Geometry check sheet. Reference: the model listing, model coordinates, mm. A direction names the side the tool comes from. Coordinates: 2 decimals unless noted, no trailing zeros. Order: outer loops, then holes, each group sorted by start corner. A loop starts at its lowest first (then second) coordinate and runs counter-clockwise, first axis right, second up. Notation, with made-up numbers: (-32, -9) - (-19, -9) arc R14 ccw to (-19, -1) - close; hole circle Ø9 at (-29, 78.25). An arc over 180 degrees is marked (long way). One line per item, written item: value. Start each with the question number.
```python
from build123d import *

# Parameters (mm, degrees)
SKETCH1_W           = 125
SKETCH1_H           = 382
BOSS_EXTRUDE1_DEPTH = 2
SKETCH2_W           = 216
SKETCH2_H           = 16
BOSS_EXTRUDE2_DEPTH = 10
SKETCH3_W           = 210
SKETCH3_H           = 10
CUT_EXTRUDE1_DEPTH  = 390.477855596


with BuildPart() as part:
    # Sketch1 → Boss-Extrude1 (new body)
    with BuildSketch(Plane(origin=(532, 0, 0), x_dir=(0, -1, 0), z_dir=(-1, 0, 0))):
        with Locations((12.5, -191)):
            Rectangle(SKETCH1_W, SKETCH1_H)
    extrude(amount=-BOSS_EXTRUDE1_DEPTH)

    # Sketch2 → Boss-Extrude2 (add)
    with BuildSketch(Plane.ZY.offset(-532)):
        with Locations((-191, 24.613657059)):
            Rectangle(SKETCH2_W, SKETCH2_H)
    extrude(amount=BOSS_EXTRUDE2_DEPTH)

    # Sketch3 → Cut-Extrude1 (cut, through all)
    with BuildSketch(Plane.ZY.offset(-522)):
        with Locations((-191, 24.613657059)):
            Rectangle(SKETCH3_W, SKETCH3_H)
    extrude(amount=-CUT_EXTRUDE1_DEPTH, mode=Mode.SUBTRACT)


solid = part.part
```
Q1. Set-up check for faces 1 (the flat face through (527, 25, -299)), 2 (the flat face through (527, 32.614, -193)), 3 (the flat face through (528, 29.614, -192)): record each of +Z, -Z, +X, -X, +Y, -Y from which the full face is reachable in a straight line by a thin tool's end or side.
Q2. Cross-section at C-C, the plane x = 524. Enter the section's corners in (y, z), and give its area (3 significant figures).
Q3. Cross-section at A-A, the plane z = -286.5. Enter the section's corners in (x, y).
Q4. Release check for a two-part mould opening along Z. For faces 4 (the flat face through (528, 19.614, -192)), 5 (the flat face through (527, 25, -83)), 6 (the flat face through (534, -12, -188)) record: released by +Z, released by -Z, zero draft, split by the parting line, or undercut.
Q5. Cross-section at D-D, the plane y = -39. Enter the section's corners in (x, z), and give its area (3 significant figures).
Q6. Material ranges on probe 1 along Y at (x, z) = (527.5, -99); probe 2 along Z at (x, y) = (525, 20); probe 3 along Y at (x, z) = (532.5, -144.5), recorded low to high.
Q7. Gauge pin test, flat ends, axial feed: P1, Ø4, axis at x = 525, y = 14.5, coming from the +Z side; P2, Ø5, axis at x = 524.5, y = 28.5, coming from the +Z side; P3, Ø10, axis at y = -13.5, z = -85, coming from the -X side; P4, Ø3, axis at x = 526, y = 22, coming from the -Z side. Record the tip position at first contact, or that the pin passes through.
Q8. Cross-section at B-B, the plane y = 26. Enter the section's corners in (x, z), and give its area (3 significant figures).
Check result:
1. face 1: -Z, -X, +Y, -Y
1. face 2: +Z, -Z, -X, +Y
1. face 3: +X, -X
2. outline: (16.61, -299) - (32.61, -299) - (32.61, -83) - (16.61, -83) - close; hole (19.61, -296) - (29.61, -296) - (29.61, -86) - (19.61, -86) - close
2. area: 1,360 mm2
3. outline: (522, 16.61) - (532, 16.61) - (532, -75) - (534, -75) - (534, 19.61) - (522, 19.61) - close; (522, 29.61) - (534, 29.61) - (534, 50) - (532, 50) - (532, 32.61) - (522, 32.61) - close
4. face 4: undercut
4. face 5: released by +Z
4. face 6: zero draft
5. outline: (532, -382) - (534, -382) - (534, 0) - (532, 0) - close
5. area: 764 mm2
6. probe 1: y = 16.61 to 19.61, 29.61 to 32.61
6. probe 2: z = -299 to -296, -86 to -83
6. probe 3: y = -75 to 19.61, 29.61 to 50
7. P1: passes through
7. P2: stops at z = -83
7. P3: stops at x = 532
7. P4: stops at z = -299
8. outline: (522, -299) - (532, -299) - (532, -382) - (534, -382) - (534, -296) - (522, -296) - close; (522, -86) - (534, -86) - (534, 0) - (532, 0) - (532, -83) - (522, -83) - close
8. area: 404 mm2
